Geometry: final body of the model. Coordinates: model frame, mm. Face numbers are marked on the shaded views. A direction names the side the tool comes from. Give positions to 0.01 mm unless a question says otherwise; leave off trailing zeros. Loops run counter-clockwise (first coordinate to the right, second up) from the corner with the lowest first, then second, coordinate; pieces in that order, holes last.
1. First-contact query: P1, Ø1.2, axis at x = -4, y = 18.5, coming from the -Z side; P2, Ø6, axis at y = 13.5, z = 5, coming from the -X side; P3, Ø3.5, axis at x = 10, z = 5, coming from the +Y side; P4, Ø1.5, axis at y = 23, z = 10.5, coming from the +X side. Flat tips, straight axial feed; report the tip coordinate or a pass-through.
2. Section A-A, the plane x = 5.9. Output: boundary loops of the cut face in (y, z), then the cut area to 3 significant figures.
3. Section C-C, the plane z = 1.5. Output: boundary loops of the cut face in (x, y), then the cut area to 3 significant figures.
4. Access query for the marked faces 1, 2 and 3. Directions: +Z, -Z, +X, -X, +Y, -Y. A direction counts if a zero-diameter tool reaches every point of the face in a straight line with its end or side. Return the directions, or none.
5. Section B-B, the plane x = -2.5. Output: boundary loops of the cut face in (y, z), then the cut area to 3 significant figures.
6. Section D-D, the plane y = 29.5. Output: boundary loops of the cut face in (x, z).
7. Material intervals for line 1 along Z through (x, y) = (-2.5, 18.8); line 2 along Y through (x, z) = (9.5, 1.75); line 3 along Y through (x, z) = (-1.5, 10.5), sorted ascending.
from build123d import *

# Parameters (mm, degrees)
EXTRUDE_1_DEPTH     = 12
SKETCH_2_R          = 2.3
EXTRUDE_2_DEPTH     = 6
SKETCH_3_R          = 2.3
EXTRUDE_3_DEPTH     = 10
CUT_EXTRUDE_1_REACH = 37.679


with BuildPart() as part:
    # 草图1 → 凸台-拉伸1 (new body)
    with BuildSketch(Plane.XY):
        Polygon((0, 0), (22, 0), (22, 18), (27, 18), (27, 20), (22, 20), (22, 21.5), (0, 21.5), (0, 20), (-5, 20), (-5, 18), (0, 18), align=None)
    extrude(amount=EXTRUDE_1_DEPTH)

    # 草图2 → 凸台-拉伸2 (add)
    with BuildSketch(Plane(origin=(0, 21.5, 0), x_dir=(1, 0, 0), z_dir=(0, 1, 0))):
        with BuildLine():
            Line((12.2, -3.5), (11.244155686, -3.5))
            ThreePointArc((11.244155686, -3.5), (0, -6), (11.244155686, -8.5))
            Line((11.244155686, -8.5), (12.2, -8.5))
            ThreePointArc((12.2, -8.5), (14.7, -6), (12.2, -3.5))
        make_face()
        with Locations(Location((5.9, -6, 0), (0, 0, 270))):
            Circle(SKETCH_2_R, mode=Mode.SUBTRACT)
    extrude(amount=EXTRUDE_2_DEPTH)

    # 草图3 → 凸台-拉伸3 (add)
    with BuildSketch(Plane(origin=(0, 21.5, 0), x_dir=(1, 0, 0), z_dir=(0, 1, 0))):
        with Locations(Location((5.9, -6, 0), (0, 0, 270))):
            Circle(SKETCH_3_R)
    extrude(amount=EXTRUDE_3_DEPTH)

    # 草图4 → 切除-拉伸1 (cut, up to next)
    with BuildSketch(Plane(origin=(0, 20, 0), x_dir=(1, 0, 0), z_dir=(0, 1, 0)), mode=Mode.PRIVATE) as cut_extrude_1_sk1:
        with BuildLine():
            Line((27, -5.2), (27, -6.8))
            Line((27, -6.8), (25.460468636, -6.8))
            ThreePointArc((25.460468636, -6.8), (23.25, -6), (25.460468636, -5.2))
            Line((25.460468636, -5.2), (27, -5.2))
        make_face()
    cut_extrude_1_tool1 = extrude(cut_extrude_1_sk1.sketch, amount=-CUT_EXTRUDE_1_REACH, mode=Mode.PRIVATE) & part.part
    # 草图4 → 切除-拉伸1 (cut, up to next)
    with BuildSketch(Plane(origin=(0, 20, 0), x_dir=(1, 0, 0), z_dir=(0, 1, 0)), mode=Mode.PRIVATE) as cut_extrude_1_sk2:
        with BuildLine():
            Line((-5, -5.2), (-5, -6.8))
            Line((-5, -6.8), (-3.460468636, -6.8))
            ThreePointArc((-3.460468636, -6.8), (-1.25, -6), (-3.460468636, -5.2))
            Line((-3.460468636, -5.2), (-5, -5.2))
        make_face()
    cut_extrude_1_tool2 = extrude(cut_extrude_1_sk2.sketch, amount=-CUT_EXTRUDE_1_REACH, mode=Mode.PRIVATE) & part.part
    add(cut_extrude_1_tool1.solids().sort_by_distance((25.055712, 20, 6))[0], mode=Mode.SUBTRACT)
    add(cut_extrude_1_tool2.solids().sort_by_distance((-3.055712, 20, 6))[0], mode=Mode.SUBTRACT)


solid = part.part
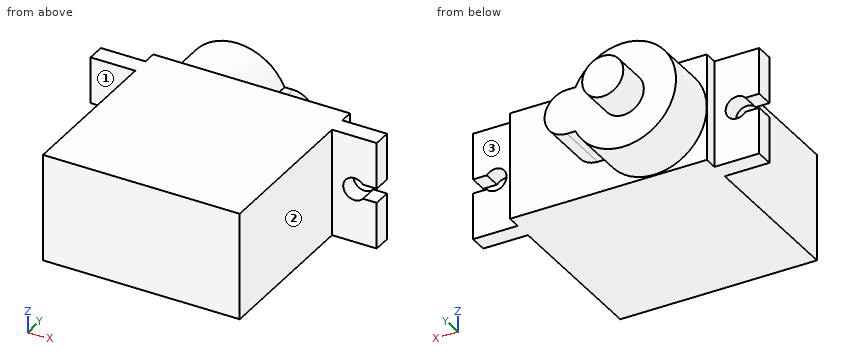
Answers below:
1. P1: stops at z = 0
1. P2: stops at x = 0
1. P3: stops at y = 27.5
1. P4: stops at x = 10.45
2. outline: (0, 0) - (21.5, 0) - (21.5, 0.1) - (27.5, 0.1) - (27.5, 3.7) - (31.5, 3.7) - (31.5, 8.3) - (27.5, 8.3) - (27.5, 11.9) - (21.5, 11.9) - (21.5, 12) - (0, 12) - close
2. area: 347 mm2
3. outline: (-5, 18) - (0, 18) - (0, 0) - (22, 0) - (22, 18) - (27, 18) - (27, 20) - (22, 20) - (22, 21.5) - (9.72, 21.5) - (9.72, 27.5) - (2.08, 27.5) - (2.08, 21.5) - (0, 21.5) - (0, 20) - (-5, 20) - close
3. area: 539 mm2
4. face 1: +Z, -Z, -X, -Y
4. face 2: +Z, -Z, +X, -Y
4. face 3: +Z, -Z, +X, +Y
5. outline: (18, 0) - (20, 0) - (20, 4.75) - (18, 4.75) - close; (18, 7.25) - (20, 7.25) - (20, 12) - (18, 12) - close
5. area: 19.0 mm2
6. outline: circle Ø4.6 at (5.9, 6)
7. line 1: z = 0 to 4.75, 7.25 to 12
7. line 2: y = 0 to 27.5
7. line 3: y = 18 to 20
